from build123d import *

# Parameters (mm, degrees)
F0_R     = 3.175
F1_DEPTH = 38.1
F2_R     = 1.5875
F3_DEPTH = 12.7
F4_R     = 0.79375
F5_DEPTH = 3.176
F6_SIZE  = 0.508


with BuildPart() as f1:
    # F0 (on Front) → F1 (new body)
    with BuildSketch(Plane.XZ):
        Circle(F0_R)
    extrude(amount=F1_DEPTH)

    # F2 (on face) → F3 (cut)
    with BuildSketch(Plane(origin=(0, 0, 0), x_dir=(-1, 0, 0), z_dir=(0, 1, 0))):
        Circle(F2_R)
    extrude(amount=-F3_DEPTH, mode=Mode.SUBTRACT)

    # F4 (on Top) → F5 (cut, through all)
    with BuildSketch(Plane.XY):
        with Locations((0, -6.35)):
            Circle(F4_R)
    extrude(amount=-F5_DEPTH, mode=Mode.SUBTRACT)

    # F6
    f6_edges = [f1.edges().sort_by_distance(p)[0] for p in [
        (-3.175, -38.1, 0),
    ]]
    chamfer(f6_edges, length=F6_SIZE)


solid = f1.part
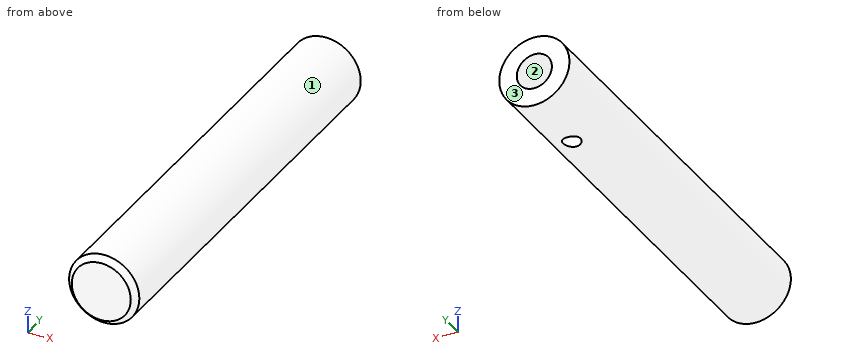
The model under review builds one solid part; all positions refer to its coordinate system, in mm. Face numbers are marked on the shaded views. Round coordinates to 2 decimals unless told otherwise and drop trailing zeros. Write each loop counter-clockwise with the first axis right and the second up, starting at its lowest first coordinate (ties: lowest second). Pieces come first, ordered by that corner, then holes. Notation, with made-up numbers: (33, 85.5) -> (50, 85.5) arc R23 ccw to (50, 104.5) -> close; hole circle Ø11 at (34.5, 13.5). An arc over 180 degrees is marked (long way). Answer as a JSON object with one key per item and string values.
1. To check wall thickness, follow line 1 along Y through (x, z) = (0, -2.2); line 2 along Z through (x, y) = (0, -9.5) (1 decimal); line 3 along Z through (x, y) = (-0.5, -2). State the ranges of each line that lie inside material, in increasing order.
Results found:
{"line 1": "y = -38.1 to -7.14, -5.56 to 0", "line 2": "z = -3.2 to -1.6, 1.6 to 3.2", "line 3": "z = -3.14 to -1.51, 1.51 to 3.14"}
2. The part is to be moulded in two halves that separate along X. For the marked faces 1, 2 and 3, say which applies: pulls with the +X half, pulls with the -X half, needs draft (parallel to the pull), parting line crosses it, or undercut.
Results found:
{"face 1": "parting line crosses it", "face 2": "undercut", "face 3": "needs draft"}
3. We need section D-D on y = -17.5. State the section outline as (x, z) points (3 decimals).
Results found:
{"outline": "circle Ø6.35 at (0, 0)"}
4. Clearance check with flat-ended pins moving along their axes: pin 1 (3 mm diameter, centred on x = 0, z = 0, fed in from +Y); pin 2 (1.5 mm diameter, centred on x = 1, y = -27, fed in from +Z); pin 3 (3 mm diameter, centred on y = -27.5, z = -2, fed in from +X). State where each tip first meets the part, or that it passes through.
Results found:
{"pin 1": "stops at y = -12.7", "pin 2": "stops at z = 3.17", "pin 3": "stops at x = 3.14"}
5. We need section A-A on x = 0. State the section outline as (y, z) points (1 decimal), and give its area (3 significant figures).
Results found:
{"outline": "(-38.1, -2.7) -> (-37.6, -3.2) -> (-7.1, -3.2) -> (-7.1, -1.6) -> (-12.7, -1.6) -> (-12.7, 1.6) -> (0, 1.6) -> (0, 3.2) -> (-37.6, 3.2) -> (-38.1, 2.7) -> close; (-5.6, -3.2) -> (0, -3.2) -> (0, -1.6) -> (-5.6, -1.6) -> close", "area": "199 mm^2"}
6. We need section B-B on z = 0. State the section outline as (x, y) points (1 decimal).
Results found:
{"outline": "(-3.2, -37.6) -> (-2.7, -38.1) -> (2.7, -38.1) -> (3.2, -37.6) -> (3.2, 0) -> (1.6, 0) -> (1.6, -12.7) -> (-1.6, -12.7) -> (-1.6, 0) -> (-3.2, 0) -> close"}
